```python
from build123d import *

# Parameters (mm, degrees)
ESQUISSE2_W             = 5.5
ESQUISSE2_H             = 0.8
ENLEV_MAT_EXTRU_1_DEPTH = 1.3
ESQUISSE3_W             = 1.5
ESQUISSE3_H             = 8
CHANFREIN1_SIZE         = 0.3


with BuildPart() as part:
    # Esquisse1 → Base-Révolution (revolve)
    with BuildSketch(Plane(origin=(0, 0, 0), x_dir=(1, 0, 0), z_dir=(0, 1, 0))):
        with BuildLine():
            Line((0, 0), (2.75, 0))
            Line((2.75, 0), (2.590995378, 1.817431149))
            ThreePointArc((2.590995378, 1.817431149), (2.52687448, 1.947455467), (2.391756438, 2))
            Line((2.391756438, 2), (0, 2))
            Line((0, 2), (0, 0))
        make_face()
    revolve(axis=Axis((0, 0, 0), (0, 0, -1)))

    # Esquisse2 → Enlev. mat.-Extru.1 (cut)
    with BuildSketch(Plane.XY.offset(-2)):
        Rectangle(ESQUISSE2_W, ESQUISSE2_H)
    extrude(amount=ENLEV_MAT_EXTRU_1_DEPTH, mode=Mode.SUBTRACT)

    # Esquisse3 → Boss.-Révol.1 (revolve)
    with BuildSketch(Plane(origin=(0, 0, 0), x_dir=(1, 0, 0), z_dir=(0, 1, 0))):
        with Locations((0.75, -4)):
            Rectangle(ESQUISSE3_W, ESQUISSE3_H)
    revolve(axis=Axis((0, 0, 0), (0, 0, 1)))

    # Chanfrein1
    chanfrein1_edges = [part.edges().sort_by_distance(p)[0] for p in [
        (-1.5, 0, 8),
    ]]
    chamfer(chanfrein1_edges, length=CHANFREIN1_SIZE)


solid = part.part
```
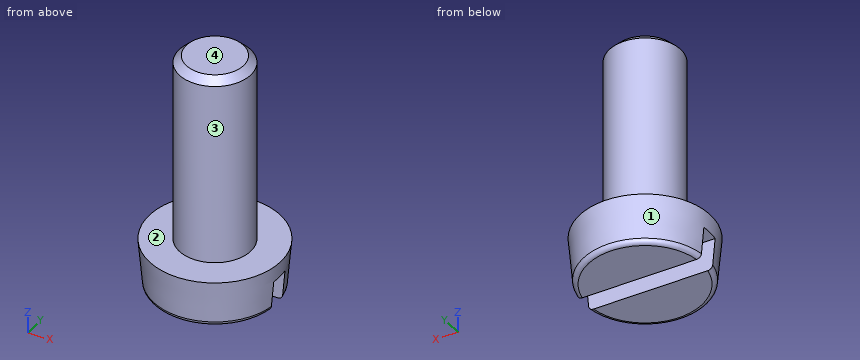
For this review, take the finished solid that the model builds, in its own axes (mm). Face numbers are marked on the shaded views. A direction names the side the tool comes from. Coordinates: 2 decimals unless noted, no trailing zeros. Order: outer loops, then holes, each group sorted by start corner. A loop starts at its lowest first (then second) coordinate and runs counter-clockwise, first axis right, second up. Notation, with made-up numbers: (18.5, 69) -> (33.5, 69) arc R13 ccw to (33.5, 73) -> close; hole circle Ø1 at (80, 63.5). An arc over 180 degrees is marked (long way). Use CSV: the item, a comma, the result in double quotes. Start each with the question number.
Item 1: We need section B-B, the plane y = 0. Give the boundary of the cut face in (x, z).
Item 2: Draft analysis for pull direction X (two halves, no side actions). For the marked faces 1 and 2, state which applies: pulls with the +X half, pulls with the -X half, needs draft (parallel to the pull), parting line crosses it, or undercut.
Item 3: Insertion check: pin 1 (2 mm diameter, centred on x = 1.5, z = 6.5, fed in from +Y); pin 2 (1 mm diameter, centred on x = 0.5, z = -1, fed in from -Y); pin 3 (2 mm diameter, centred on y = 0, z = 6, fed in from +X). Each pin has a flat end and moves straight along its axis. Give the tip position at first contact, or say it passes through.
Item 4: Wall thickness on probe 1 along Z at (x, y) = (-0.85, -0.1); probe 2 along Z at (x, y) = (1.25, 1.5); probe 3 along Y at (x, z) = (-0.1, -1): over which ranges is each line inside the solid? List them lowest first.
Item 5: For the marked faces 3 and 4, list the 3-axis set-ups (+Z, -Z, +X, -X, +Y, -Y) from which the entire face can be reached by the end or side of a thin tool; tool diameter is ignored.
Item 6: We need section C-C, the plane z = 3.5. Give the boundary of the cut face in (x, y), then the cut area to 3 significant figures.
Item 7: We need section A-A, the plane x = 0. Give the boundary of the cut face in (y, z), then the cut area to 3 significant figures.
Derived:
1,outline,"(-2.75, 0) -> (-2.69, -0.7) -> (2.69, -0.7) -> (2.75, 0) -> (1.5, 0) -> (1.5, 7.7) -> (1.2, 8) -> (-1.2, 8) -> (-1.5, 7.7) -> (-1.5, 0) -> close"
2,face 1,"parting line crosses it"
2,face 2,"needs draft"
3,pin 1,"stops at y = 1.41"
3,pin 2,"stops at y = -2.69"
3,pin 3,"stops at x = 1.5"
4,probe 1,"z = -0.7 to 8"
4,probe 2,"z = -2 to 0"
4,probe 3,"y = -2.66 to -0.4, 0.4 to 2.66"
5,face 3,"+Z"
5,face 4,"+Z, +X, -X, +Y, -Y"
6,outline,"circle Ø3 at (0, 0)"
6,area,"7.07 mm^2"
7,outline,"(-2.75, 0) -> (-2.59, -1.82) arc R0.2 ccw to (-2.39, -2) -> (-0.4, -2) -> (-0.4, -0.7) -> (0.4, -0.7) -> (0.4, -2) -> (2.39, -2) arc R0.2 ccw to (2.59, -1.82) -> (2.75, 0) -> (1.5, 0) -> (1.5, 7.7) -> (1.2, 8) -> (-1.2, 8) -> (-1.5, 7.7) -> (-1.5, 0) -> close"
7,area,"33.5 mm^2"
